Geometry check sheet. Reference: the model listing, model coordinates, mm. A direction names the side the tool comes from. Coordinates: 2 decimals unless noted, no trailing zeros. Order: outer loops, then holes, each group sorted by start corner. A loop starts at its lowest first (then second) coordinate and runs counter-clockwise, first axis right, second up. Notation, with made-up numbers: M -19.5,31.25 L -4.5,31.25 A21 cw -4.5,58.25 Z; hole C 12.5,-34.75 d8. An arc over 180 degrees is marked long. Use CSV: the item, a comma, the result in double quotes. Start each with the question number.
Autodesk Inventor part; units mm, degrees
ref_plane "YZ Plane" through (0, 0, 0) normal (1, 0, 0) x (0, 1, 0)
ref_plane "XZ Plane" through (0, 0, 0) normal (0, 1, 0) x (-1, 0, 0)
ref_plane "XY Plane" through (0, 0, 0) normal (0, 0, 1) x (1, 0, 0)
sketch "Skizze1" plane through (0, 0, 0) normal (0, 0, 1) x (1, 0, 0)
  line L0 (-68.016, 1.808) -> (67.584, 1.808)
  line L1 (67.584, 1.808) -> (67.584, -2.192)
  line L2 (67.584, -2.192) -> (-68.016, -2.192)
  line L3 (-68.016, -2.192) -> (-68.016, 1.808)
  line L4 (-68.016, 1.808) -> (67.584, -2.192) construction
  line L5 (67.584, 1.808) -> (-68.016, -2.192) construction
  point P0 (0, 0)
  point P1 (-0.216, -0.192)
  point P2 (-0.216, -0.192)
  dimension "d0" = 135.6
  dimension "d1" = 4
extrude "Extrusion1" add sketch "Skizze1" along normal mid plane 3.25
ref_plane "Arbeitsebene1" through (-68.016, -0.192, 1.625) normal (0, -1, 0) x (1, 0, 0)
sketch "Skizze2" plane through (-68.016, -0.192, 1.625) normal (0, -1, 0) x (1, 0, 0)
  line L0 (0, -3.25) -> (0, 0)
  line L1 (0, -3.25) -> (135.6, -3.25)
  line L2 (0, 0) -> (2.85, 0)
  line L3 (2.85, 0) -> (2.85, -3.25)
  line L4 (2.85, -3.25) -> (0, -3.25)
  line L5 (0, -3.25) -> (0, 0)
  line L6 (0, 0) -> (0, 1.75)
  line L7 (0, 1.75) -> (2.85, 0)
  line L8 (135.6, -3.25) -> (135.6, 0)
  line L9 (135.6, 0) -> (132.75, 0)
  line L10 (132.75, 0) -> (132.75, -3.25)
  line L11 (132.75, -3.25) -> (135.6, -3.25)
  line L12 (135.6, -3.25) -> (135.6, 0)
  line L13 (135.6, 0) -> (135.6, 1.75)
  line L14 (135.6, 1.75) -> (132.75, 0)
  point P0 (68.016, -1.625)
  dimension "d4" = 2.85
  dimension "d5" = 1.75
  dimension "d6" = 2.85
extrude "Extrusion2" add sketch "Skizze2" along normal mid plane 19.7
sketch "Skizze3" plane through (0, 0, 1.625) normal (0, 0, 1) x (1, 0, 0)
  circle A0 centre (0, 0) radius 16
  dimension "d9" = 32
extrude "Extrusion3" cut sketch "Skizze3" against normal through all
sketch "Skizze4" plane through (0, 0, -1.625) normal (0, 0, -1) x (-1, 0, 0)
  line L0 (0.0777, -0.1628) -> (6.2277, -0.1628) construction
  circle A0 centre (0.0009, -0.1935) radius 14.07
  circle A1 centre (0.0009, -0.1935) radius 17.07
  line L1 (-24.5991, -8.0335) -> (24.6009, -8.0335)
  point P0 (-17.0691, -0.1935)
  point P1 (17.0709, -0.1935)
  point P2 (11.6842, -8.0335)
  point P3 (15.164, -8.0335)
  point P4 (-15.1622, -8.0335)
  point P5 (-11.6824, -8.0335)
  dimension "d27" = 3
  dimension "d28" = 28.14
  dimension "d29" = 7.84
extrude "Extrusion4" add sketch "Skizze4" against normal blind 6.5 contours A0 L1 A1 picked at (15.9061, 1.1659)
sketch "Skizze7" plane through (0, 0, 1.625) normal (0, 0, 1) x (1, 0, 0)
  line L0 (-65.166, 1.808) -> (-16.9531, 1.808)
  line L1 (-16.9535, -2.192) -> (-65.166, -2.192)
  line L2 (-16.9531, 1.808) -> (-61.9531, 1.808)
  line L3 (-61.9531, 1.808) -> (-61.9531, -2.192)
  line L4 (-61.9531, -2.192) -> (-16.9531, -2.192)
  line L5 (-16.9531, -2.192) -> (-16.9531, 1.808)
  line L6 (16.9514, 1.808) -> (64.734, 1.808)
  line L7 (64.734, -2.192) -> (16.9517, -2.192)
  line L8 (16.9514, 1.808) -> (61.9514, 1.808)
  line L9 (61.9514, 1.808) -> (61.9514, -2.192)
  line L10 (61.9514, -2.192) -> (16.9514, -2.192)
  line L11 (16.9514, -2.192) -> (16.9514, 1.808)
  point P0 (0, 0)
  point P1 (16.9517, -2.192)
  dimension "d30" = 45
  dimension "d31" = 45
extrude "Extrusion7" add sketch "Skizze7" along normal blind 3.25
sketch "Skizze8" plane through (-65.166, -2.192, -1.625) normal (0, -1, 0) x (1, 0, 0)
  line L0 (48.2128, 6.5) -> (3.2128, 6.5)
  line L1 (48.2128, 6.5) -> (48.2128, 0)
  line L2 (3.2128, 6.5) -> (48.2128, 6.5)
  line L3 (48.2128, 6.5) -> (48.2128, 3.25)
  line L4 (48.2128, 3.25) -> (3.2128, 3.25)
  line L5 (3.2128, 3.25) -> (3.2128, 6.5)
  line L6 (127.1173, 3.25) -> (127.1173, 6.5)
  line L7 (82.1173, 6.5) -> (82.1173, 0)
  line L8 (127.1173, 6.5) -> (82.1173, 6.5)
  line L9 (82.1173, 6.5) -> (82.1173, 3.25)
  line L10 (82.1173, 3.25) -> (127.1173, 3.25)
  line L11 (127.1173, 3.25) -> (127.1173, 6.5)
  line L12 (82.1173, 6.5) -> (127.1173, 3.25)
  line L13 (50.002, 6.5) -> (48.2125, 6.5)
  line L14 (48.2125, 6.5) -> (3.2128, 3.25)
  point P0 (65.166, 1.625)
extrude "Extrusion8" cut sketch "Skizze8" against normal through all contours L14 L5 L0 | L12 L8 L6
properties part number "2024_08_23_Holder_GL25"
1) Section check C-C on x = -20. Record the boundary of the cut face in (y, z) (3 decimals), then the cut area to 3 significant figures.
2) Section check A-A on y = -0.25. Record the boundary of the cut face in (x, z) (3 decimals), then the cut area to 3 significant figures.
3) Section check D-D on x = 34. Record the boundary of the cut face in (y, z) (3 decimals), then the cut area to 3 significant figures.
4) Material ranges on line 1 along X through (y, z) = (-1, 0); line 2 along X through (y, z) = (-6, 2.25); line 3 along Y through (x, z) = (26, 4), recorded low to high.
5) Draft check along X on faces 6 (the face through (63, 0, 1.625)), 7 (the face through (-67, -10.042, 0)), 8 (the face through (67.584, 0, 1)), 9 (the face through (39.136, -0.22, 3.273)). Enter one of: +X half, -X half, draft (parallel to the pull), parting line (faces both ways), or undercut.
6) Section check B-B on y = 8.25. Record the boundary of the cut face in (x, z) (3 decimals).
7) Set-up check for faces 1 (the face through (-41, 1.808, 1)), 2 (the face through (64.734, -6, 0)), 3 (the face through (-66.61, -0.05, 2.51)), 4 (the face through (-67, 9.658, 0)), 5 (the face through (66, 9.658, 0)): record each of +Z, -Z, +X, -X, +Y, -Y from which the full face is reachable in a straight line by a thin tool's end or side.
8) Gauge pin test, flat ends, axial feed: P1, Ø3, axis at x = 45.5, z = 0.5, coming from the -Y side; P2, Ø1.4, axis at x = -66, z = 0, coming from the +Y side; P3, Ø3, axis at x = 13.5, z = 1, coming from the -Y side; P4, Ø1.5, axis at x = -30.5, y = 3.5, coming from the -Z side. Record the tip position at first contact, or that the pin passes through.
Results are:
1,outline,"M -2.192,-1.625 L 1.808,-1.625 L 1.808,4.655 L -2.192,4.655 Z"
1,area,"25.1 mm²"
2,outline,"M -68.016,-1.625 L -14.071,-1.625 L -14.071,4.875 L -16.953,4.875 L -61.953,1.625 L -65.166,1.625 L -68.016,3.375 Z; M 14.069,-1.625 L 67.584,-1.625 L 67.584,3.375 L 64.734,1.625 L 61.951,1.625 L 16.951,4.875 L 14.069,4.875 Z"
2,area,"519 mm²"
3,outline,"M -2.192,-1.625 L 1.808,-1.625 L 1.808,3.644 L -2.192,3.644 Z"
3,area,"21.1 mm²"
4,line 1,"x = -68.02 to -14.05, 14.05 to 67.58"
4,line 2,"x = -68.02 to -66.18, -16.05 to -12.82, 12.82 to 16.05, 65.75 to 67.58"
4,line 3,"y = -2.19 to 1.81"
5,face 6,"undercut"
5,face 7,"draft"
5,face 8,"+X half"
5,face 9,"undercut"
6,outline,"M -68.016,-1.625 L -65.166,-1.625 L -65.166,1.625 L -68.016,3.375 Z; M -14.836,-1.625 L -11.256,-1.625 L -11.256,4.875 L -14.836,4.875 Z; M 11.254,-1.625 L 14.835,-1.625 L 14.835,4.875 L 11.254,4.875 Z; M 64.734,-1.625 L 67.584,-1.625 L 67.584,3.375 L 64.734,1.625 Z"
7,face 1,"+Z, -Z, +Y"
7,face 2,"+Z, -Z, -Y"
7,face 3,"+Z, +Y, -Y"
7,face 4,"+Z, -Z, -X, +Y"
7,face 5,"+Z, -Z, +X, +Y"
8,P1,"stops at y = -2.19"
8,P2,"stops at y = 9.66"
8,P3,"stops at y = -8.03"
8,P4,"passes through"
